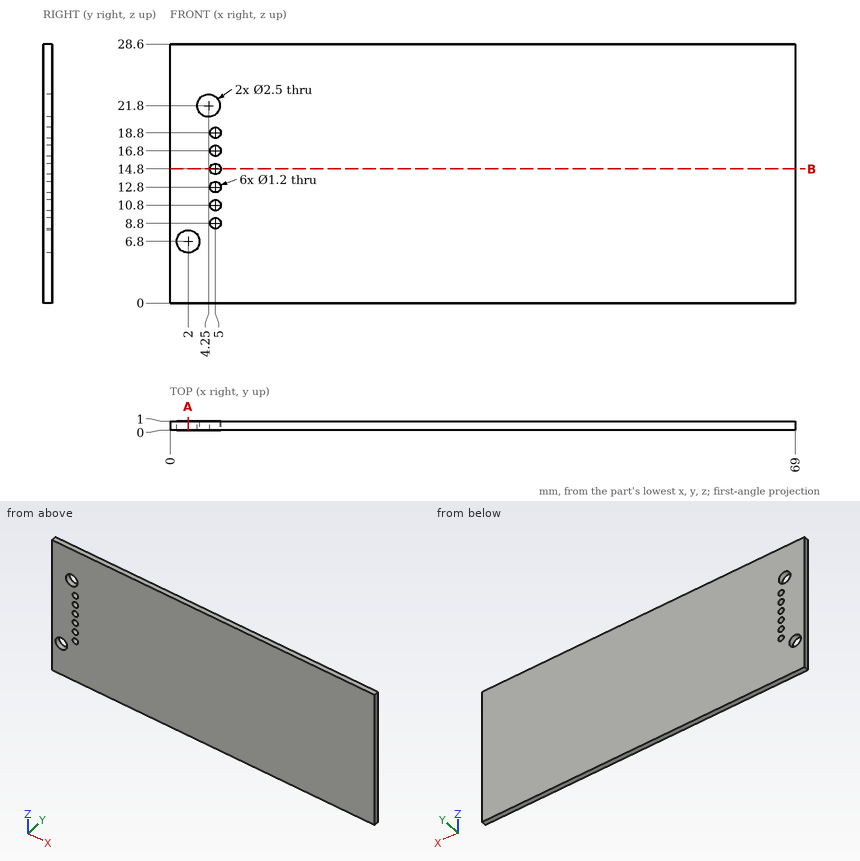
Design review of the part shown in the three views and the two pictorial views. Dimensions are in mm from the part's minimum x, y and z. Give positions to 0.01 mm unless a question says otherwise; leave off trailing zeros. Order: outer loops, then holes, each group sorted by start corner. A loop starts at its lowest first (then second) coordinate and runs counter-clockwise, first axis right, second up. Notation, with made-up numbers: (52.25, -2.75) -> (107.25, -2.75) arc R31 cw to (107.25, 28.25) -> close; hole circle Ø9 at (69.25, -36). An arc over 180 degrees is marked (long way). Write each question's results on one line, items separated by ' | '. Start each with the question number.
Q1. Add section A-A on x = 2. Give the boundary of the cut face in (y, z), and give its area (3 significant figures).
Q2. Add section B-B on z = 14.8. Give the boundary of the cut face in (x, y), and give its area (3 significant figures).
Q3. Wall thickness on L1, parallel to Z at x = 2, y = 0.6; L2, parallel to Z at x = 4.25, y = 0.5; L3, parallel to X at y = 0.35, z = 6.75: over which ranges is each line inside the solid? List them lowest first. Write a range as from..to.
Q4. For pin 1 (3 mm diameter, centred on x = 30.5, z = 8.5, fed in from -Y), flat-tipped, find the tip position at first contact; note if it passes through.
Found:
1) outline: (0, 0) -> (1, 0) -> (1, 5.55) -> (0, 5.55) -> close; (0, 8.05) -> (1, 8.05) -> (1, 28.6) -> (0, 28.6) -> close | area: 26.1 mm2
2) outline: (0, 0) -> (4.4, 0) -> (4.4, 1) -> (0, 1) -> close; (5.6, 0) -> (69, 0) -> (69, 1) -> (5.6, 1) -> close | area: 67.8 mm2
3) L1: z = 0..5.55, 8.05..28.6 | L2: z = 0..20.55, 23.05..28.6 | L3: x = 0..0.75, 3.25..69
4) pin 1: stops at y = 0
